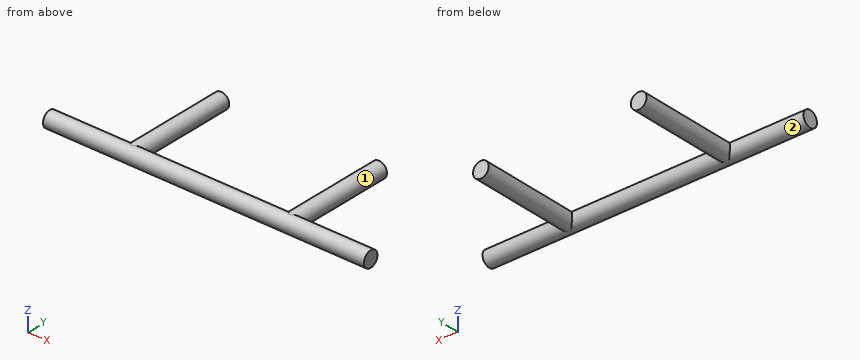
Autodesk Inventor part; units mm, degrees
ref_plane "XY Plane" through (0, 0, 0) normal (0, 0, 1) x (1, 0, 0)
sketch "Skizze1" plane through (0, 0, 0) normal (0, 0, 1) x (1, 0, 0)
  line L0 (-30.5, 0) -> (30.5, 0)
  line L1 (30.5, 0) -> (30.5, 1.5)
  line L2 (30.5, 1.5) -> (-30.5, 1.5)
  line L3 (-30.5, 1.5) -> (-30.5, 0)
  line L4 (-42.7, 0) -> (42.7, 0)
  line L5 (0, 1.8) -> (0, -0.3)
  point P0 (0, 0)
  dimension "d0" = 61
  dimension "d1" = 1.5
  dimension "d2" = 0
  dimension "d10" = 30.5
revolve "Umdrehung1" add sketch "Skizze1" angle 360 about axis through (0, 0, 0) along (1, 0, 0)
sketch "Skizze2" plane through (0, 0, 0) normal (0, 1, 0) x (-1, 0, 0)
  circle A0 centre (15, 0) radius 1.5
  circle A1 centre (-15, 0) radius 1.5
  point P0 (0, 0)
  dimension "d4" = 3
  dimension "d5" = 3
  dimension "d6" = 15
  dimension "d7" = 15
extrude "Extrusion1" add sketch "Skizze2" along normal blind 20
properties part number "Adaptation_2"
Check sheet for the modelled part. Datum: model origin and axes. Units: mm. Face numbers are marked on the shaded views. A direction names the side the tool comes from. Round coordinates to 2 decimals unless told otherwise and drop trailing zeros. Order: outer loops, then holes, each group sorted by start corner. A loop starts at its lowest first (then second) coordinate and runs counter-clockwise, first axis right, second up. Notation, with made-up numbers: (5, -9) - (42, -9) arc R16 cw to (42, 7) - close; hole circle Ø6 at (-32, 56.25). An arc over 180 degrees is marked (long way). Write item = value, one per line.
Q1. Section check C-C (x = 20). Record the boundary of the cut face in (y, z).
Computed:
outline = circle Ø3 at (0, 0)
Q2. Section check A-A (z = -0.95). Record the boundary of the cut face in (x, y).
Computed:
outline = (-30.5, -1.16) - (30.5, -1.16) - (30.5, 1.16) - (16.16, 1.16) - (16.16, 20) - (13.84, 20) - (13.84, 1.16) - (-13.84, 1.16) - (-13.84, 20) - (-16.16, 20) - (-16.16, 1.16) - (-30.5, 1.16) - close
Q3. Thickness scan on line 1 along X through (y, z) = (15.5, -0.05); line 2 along X through (y, z) = (17.5, 0.45); line 3 along Y through (x, z) = (1, 0.2). Record the ranges inside material, lowest first.
Computed:
line_1 = -16.5 to -13.5, 13.5 to 16.5
line_2 = -16.43 to -13.57, 13.57 to 16.43
line_3 = -1.49 to 1.49
Q4. Section check B-B (y = 7.5). Record the boundary of the cut face in (x, z).
Computed:
outline = circle Ø3 at (-15, 0); circle Ø3 at (15, 0)
Q5. Tool access check on the marked faces 1 and 2. Record the directions out of +Z, -Z, +X, -X, +Y, -Y that give a thin tool (end or side, any length) a straight path to the whole face; none if there is none.
Computed:
face_1 = +Y
face_2 = none
